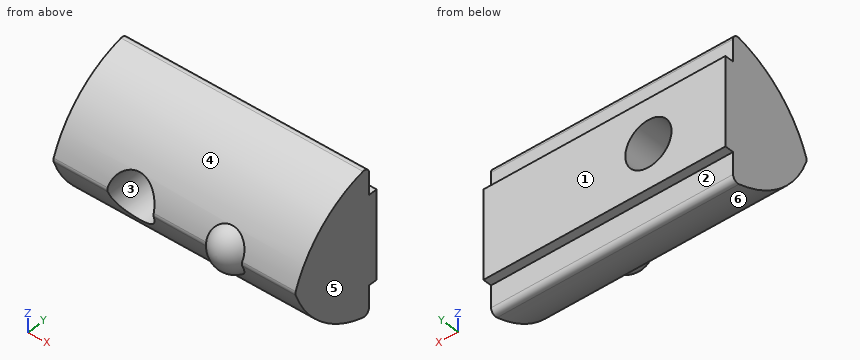
```python
from build123d import *

# Parameters (mm, degrees)
DODANIE_WYCI_GNI_CIE1_DEPTH = 11
ZAOKR_GLENIE1_R             = 0.5
OTW_R_GWINTOWANY_M51_D      = 4.2


with BuildPart() as part:
    # Szkic1 → Dodanie-wyciągnięcie1 (new, symmetric)
    with BuildSketch(Plane(origin=(0, 0, 0), x_dir=(0, 0, -1), z_dir=(1, 0, 0))):
        with BuildLine():
            Line((-4, 0), (4, 0))
            Line((4, 0), (4, -0.8))
            Line((4, -0.8), (6.6, -0.8))
            ThreePointArc((6.6, -0.8), (4.348518436, -5.548730088), (0, -8.5))
            ThreePointArc((0, -8.5), (-4.348518436, -5.548730088), (-6.6, -0.8))
            Line((-6.6, -0.8), (-4, -0.8))
            Line((-4, -0.8), (-4, 0))
        make_face()
    extrude(amount=DODANIE_WYCI_GNI_CIE1_DEPTH, both=True)

    # Zaokrąglenie1
    zaokr_glenie1_edges = [part.edges().sort_by_distance(p)[0] for p in [
        (0, -0.8, -6.6),
        (0, -8.5, 0),
        (0, -0.8, 6.6),
    ]]
    fillet(zaokr_glenie1_edges, radius=ZAOKR_GLENIE1_R)

    # Otwór gwintowany M51 (through all)
    with Locations(Plane(origin=(0, 0, 0), x_dir=(1, 0, 0), z_dir=(0, 1, 0))):
        with Locations((-4, 0)):
            Hole(OTW_R_GWINTOWANY_M51_D / 2)

    # Szkic4 → Obrót1 (revolve)
    with BuildSketch(Plane.ZY.offset(-4.5)):
        with BuildLine():
            Line((0, -5.3), (0, -9.3))
            ThreePointArc((0, -9.3), (2, -7.3), (0, -5.3))
        make_face()
    revolve(axis=Axis((4.5, -5.3, 0), (0, -1, 0)))


solid = part.part
```
Verification items for the finished model (mm, model axes). Face numbers are marked on the shaded views. A direction names the side the tool comes from. Coordinates: 2 decimals unless noted, no trailing zeros. Loops run counter-clockwise (first coordinate to the right, second up) from the corner with the lowest first, then second, coordinate; pieces in that order, holes last. Notation, with made-up numbers: (-18, 7.5) -> (-13, 7.5) arc R22 cw to (-13, 41.5) -> close; hole circle Ø10 at (62, -39). An arc over 180 degrees is marked (long way). Put each result on its own line as item: value.
1. Section check B-B, the plane x = -3.75. Record the boundary of the cut face in (y, z), then the cut area to 3 significant figures.
Result set:
outline: (-7.5, -2.09) arc R10 ccw to (-1.42, -6.47) arc R0.5 ccw to (-0.8, -5.98) -> (-0.8, -4) -> (0, -4) -> (0, -2.09) -> close; (-7.5, 2.09) -> (0, 2.09) -> (0, 4) -> (-0.8, 4) -> (-0.8, 5.98) arc R0.5 ccw to (-1.42, 6.47) arc R10 ccw to start
area: 42.4 mm^2
2. Section check C-C, the plane z = -5. Record the boundary of the cut face in (x, y), then the cut area to 3 significant figures.
Result set:
outline: (-11, -4.7) -> (11, -4.7) -> (11, -0.8) -> (-11, -0.8) -> close
area: 85.8 mm^2
3. Thickness scan on line 1 (Z direction, x = -4, y = -2.25); line 2 (Z direction, x = -2.25, y = -4.5); line 3 (X direction, y = -5, z = -0.75). Record the ranges inside material, lowest first.
Result set:
line 1: z = -6.23 to -2.1, 2.1 to 6.23
line 2: z = -5.13 to -1.16, 1.16 to 5.13
line 3: x = -11 to -5.96, -2.04 to 11
4. Mould release check, pull along Z, two halves, no side actions. Record for the marked faces 3, 4, 5 and 6: pulls with the +Z half, pulls with the -Z half, needs draft (parallel to the pull), parting line crosses it, or undercut.
Result set:
face 3: undercut
face 4: pulls with the +Z half
face 5: needs draft
face 6: pulls with the -Z half
5. Tool access check on the marked faces 1 and 2. Record the directions out of +Z, -Z, +X, -X, +Y, -Y that give a thin tool (end or side, any length) a straight path to the whole face; none if there is none.
Result set:
face 1: +Z, -Z, +X, -X, +Y
face 2: -Z, +X, -X, +Y
6. Section check D-D, the plane y = -5.25. Record the boundary of the cut face in (x, z), then the cut area to 3 significant figures.
Result set:
outline: (-11, -4.59) -> (11, -4.59) -> (11, 4.59) -> (-11, 4.59) -> close; hole circle Ø4.2 at (-4, 0)
area: 188 mm^2
7. Gauge pin test, flat ends, axial feed: P1, Ø4, axis at x = 8, y = -7.5, coming from the -Z side; P2, Ø4, axis at x = 2, z = -5, coming from the -Y side; P3, Ø6, axis at x = 0, z = 0, coming from the -Y side. Record the tip position at first contact, or that the pin passes through.
Result set:
P1: stops at z = -4.39
P2: stops at y = -6.85
P3: stops at y = -8.62
8. Section check A-A, the plane y = -0.25. Record the boundary of the cut face in (x, z), then the cut area to 3 significant figures.
Result set:
outline: (-11, -4) -> (11, -4) -> (11, 4) -> (-11, 4) -> close; hole circle Ø4.2 at (-4, 0)
area: 162 mm^2
